```python
from build123d import *

# Parameters (mm, degrees)
SKETCH2_R           = 6
BOSS_EXTRUDE1_DEPTH = 36
SKETCH3_R           = 4
CUT_EXTRUDE1_DEPTH  = 2
SKETCH4_R           = 0.5
BOSS_EXTRUDE4_DEPTH = 3


with BuildPart() as part:
    # Sketch2 → Boss-Extrude1 (new body)
    with BuildSketch(Plane(origin=(0, 0, 0), x_dir=(0, 0, -1), z_dir=(1, 0, 0))):
        Circle(SKETCH2_R)
    extrude(amount=BOSS_EXTRUDE1_DEPTH)

    # Sketch3 → Cut-Extrude1 (cut)
    with BuildSketch(Plane(origin=(36, 0, 0), x_dir=(0, 0, -1), z_dir=(1, 0, 0))):
        Circle(SKETCH3_R)
    extrude(amount=-CUT_EXTRUDE1_DEPTH, mode=Mode.SUBTRACT)

    # Sketch4 → Boss-Extrude4 (add)
    with BuildSketch(Plane(origin=(0, 0, 0), x_dir=(0, 0, -1), z_dir=(1, 0, 0))):
        with Locations((0.51, 0)):
            Circle(SKETCH4_R)
        with Locations(Location((-0.51, 0, 0), (0, 0, 180))):
            Circle(SKETCH4_R)
    extrude(amount=-BOSS_EXTRUDE4_DEPTH)


solid = part.part
```
The listing builds one solid part. Answer for the finished solid, in the listing's coordinates (mm). A direction names the side the tool comes from. Coordinates: 2 decimals unless noted, no trailing zeros. Write each loop counter-clockwise with the first axis right and the second up, starting at its lowest first coordinate (ties: lowest second). Pieces come first, ordered by that corner, then holes. Notation, with made-up numbers: M 46.5,-21.5 L 74.5,-21.5 A14 cw 74.5,-0.5 Z; hole C 35,-16 d1. An arc over 180 degrees is marked long. Use a Markdown table: item, result. Add a question column.
1. Section C-C (x = 2) is taken. Give the vertices of the cut face in (y, z).
2. Given P1, Ø2.5, axis at y = -1, z = 1, coming from the +X side; P2, Ø4, axis at y = -5, z = -4.5, coming from the -X side; P3, Ø2, axis at x = 12, z = -1.5, coming from the -Y side, each flat-ended and moving along its own axis, determine where each tip first touches the part or whether it passes through.
3. Which of the six approach directions +Z, -Z, +X, -X, +Y, -Y give full straight-line access (tool end or side, diameter ignored) to faces 4 (the cylindrical face through (35.014, -3.905, 0.867)), 5 (the flat face through (36, -3.92, 1.42))?
4. For a pull along Z with two mould halves and no side action, classify faces 1 (the flat face through (34, 0, 0)), 2 (the flat face through (-3, 0, 0.5)), 3 (the cylindrical face through (18, 0, 6)) as +Z half, -Z half, draft (parallel to the pull), parting line (faces both ways), or undercut.
5. Straight lines are drawn through the part: line 1 along Y through (x, z) = (35.55, 0); line 2 along X through (y, z) = (4.5, 2.5); line 3 along X through (y, z) = (-0.25, -3.75). For each, find the intervals that lie inside material, in ascending order. Write a range as [from, to].
6. Section B-B (z = 0.51) is taken. Give the vertices of the cut face in (x, y), plus the area to 3 significant figures.
7. Section A-A (y = 3.25) is taken. Give the vertices of the cut face in (x, z).
8. Section D-D (z = 2.5) is taken. Give the vertices of the cut face in (x, y).
Data:
| question | item | result |
|---|---|---|
| 1 | outline | C 0,0 d12 |
| 2 | P1 | stops at x = 34 |
| 2 | P2 | stops at x = 0 |
| 2 | P3 | stops at y = -5.98 |
| 3 | face 4 | +X |
| 3 | face 5 | +Z, -Z, +X, +Y, -Y |
| 4 | face 1 | undercut |
| 4 | face 2 | draft |
| 4 | face 3 | parting line |
| 5 | line 1 | y = [-6, -4], [4, 6] |
| 5 | line 2 | x = [0, 36] |
| 5 | line 3 | x = [0, 34] |
| 6 | outline | M -3,-0.5 L 0,-0.5 L 0,-5.98 L 36,-5.98 L 36,-3.97 L 34,-3.97 L 34,3.97 L 36,3.97 L 36,5.98 L 0,5.98 L 0,0.5 L -3,0.5 Z |
| 6 | area | 418 mm2 |
| 7 | outline | M 0,-5.04 L 36,-5.04 L 36,-2.33 L 34,-2.33 L 34,2.33 L 36,2.33 L 36,5.04 L 0,5.04 Z |
| 8 | outline | M 0,-5.45 L 36,-5.45 L 36,-3.12 L 34,-3.12 L 34,3.12 L 36,3.12 L 36,5.45 L 0,5.45 Z |
